```python
from build123d import *

# Parameters (mm, degrees)
SKETCH1_R           = 4.5
BOSS_EXTRUDE1_DEPTH = 55
SKETCH2_W           = 1
SKETCH2_H           = 1.8
BOSS_EXTRUDE2_DEPTH = 6
SKETCH3_W           = 1.2
SKETCH3_H           = 2
CUT_EXTRUDE1_DEPTH  = 6
FILLET1_R           = 2.5


with BuildPart() as part:
    # Sketch1 → Boss-Extrude1 (new body)
    with BuildSketch(Plane(origin=(0, 0, 0), x_dir=(1, 0, 0), z_dir=(0, 1, 0))):
        with Locations(Location((0, 0, 0), (0, 0, 270))):
            Circle(SKETCH1_R)
    extrude(amount=BOSS_EXTRUDE1_DEPTH)

    # Sketch2 → Boss-Extrude2 (add)
    with BuildSketch(Plane(origin=(0, 55, 0), x_dir=(1, 0, 0), z_dir=(0, 1, 0))):
        Rectangle(SKETCH2_W, SKETCH2_H)
    extrude(amount=BOSS_EXTRUDE2_DEPTH)

    # Sketch3 → Cut-Extrude1 (cut)
    with BuildSketch(Plane.XZ):
        Rectangle(SKETCH3_W, SKETCH3_H)
    extrude(amount=-CUT_EXTRUDE1_DEPTH, mode=Mode.SUBTRACT)

    # Fillet1
    fillet1_edges = [part.edges().sort_by_distance(p)[0] for p in [
        (0, 0, -4.5),
        (0, 55, -4.5),
    ]]
    fillet(fillet1_edges, radius=FILLET1_R)


solid = part.part
```
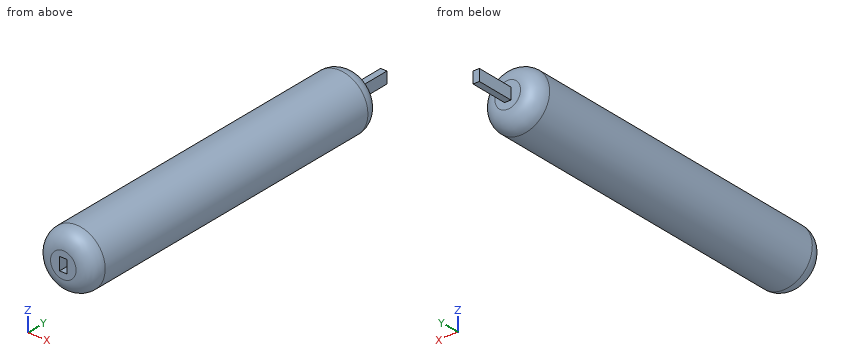
The listing builds one solid part. Answer for the finished solid, in the listing's coordinates (mm). Give positions to 0.01 mm unless a question says otherwise; leave off trailing zeros. Loops run counter-clockwise (first coordinate to the right, second up) from the corner with the lowest first, then second, coordinate; pieces in that order, holes last. Notation, with made-up numbers: M 10,-18 L 64,-18 A16 cw 64,-12 Z; hole C -7.75,-32.75 d4. An arc over 180 degrees is marked long. One line per item, written item: value.
Q1. Find the intervals of material crossed by line 1 (Z direction, x = -3.25, y = 28.5); line 2 (Y direction, x = 2.25, z = 1.25); line 3 (X direction, y = 3, z = 1.75), in increasing order. Write a range as from..to.
Working result:
line 1: z = -3.11..3.11
line 2: y = 0.07..54.93
line 3: x = -4.15..4.15
Q2. A cutting plane is placed at A-A on y = 10. Determine the outline of the cut face in (x, z), then the cut area to 3 significant figures.
Working result:
outline: C 0,0 d9
area: 63.6 mm^2
Q3. Flat-ended cylindrical pins translate along their axes: P1, Ø1.5, axis at x = 1, z = -2.5, coming from the +Y side; P2, Ø0.6, axis at x = 0, z = 0.5, coming from the -Y side; P3, Ø4, axis at x = -3.5, y = 7, coming from the -Z side. Find the tip coordinate at first contact, or state that the pin passes through.
Working result:
P1: stops at y = 55
P2: stops at y = 6
P3: stops at z = -4.24
